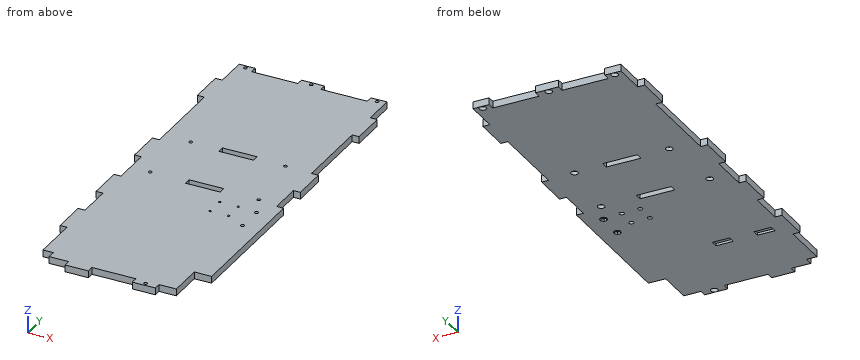
```python
from build123d import *

# Parameters (mm, degrees)
BOSS_EXTRU_1_DEPTH      = 6
ESQUISSE2_R             = 1.5
ESQUISSE2_W             = 30
ESQUISSE2_H             = 6
ENL_V_MAT_EXTRU_1_DEPTH = 226.720818795
ESQUISSE5_R             = 2.995
ENL_V_MAT_EXTRU_2_DEPTH = 3
ESQUISSE6_R             = 1.005
ENL_V_MAT_EXTRU_3_DEPTH = 226.720818795
ESQUISSE7_R             = 2
ENL_V_MAT_EXTRU_4_DEPTH = 2
ESQUISSE8_W             = 15
ESQUISSE8_H             = 30
ESQUISSE8_W_2           = 9
ESQUISSE8_H_2           = 7
ENL_V_MAT_EXTRU_5_DEPTH = 226.720818795
ESQUISSE13_R            = 1.6
ENL_V_MAT_EXTRU_7_DEPTH = 6
ESQUISSE14_W            = 15
ESQUISSE14_H            = 6
ESQUISSE14_R            = 1.6
ENL_V_MAT_EXTRU_8_DEPTH = 2


with BuildPart() as part:
    # Esquisse1 → Boss.-Extru.1 (new body)
    with BuildSketch(Plane.XY):
        Polygon((-67.628238976, -36.290343107), (-67.628238976, -70.290343107), (-73.628238976, -70.290343107), (-73.628238976, -100.290343107), (-67.628238976, -100.290343107), (-67.628238976, -130.290343107), (-73.628238976, -130.290343107), (-73.628238976, -160.290343107), (-67.628238976, -160.290343107), (-67.628238976, -207.290343107), (-41.628238976, -207.290343107), (-41.628238976, -213.290343107), (-21.628238976, -213.290343107), (-21.628238976, -207.290343107), (16.371761024, -207.290343107), (16.371761024, -213.290343107), (36.371761024, -213.290343107), (36.371761024, -207.290343107), (66.371761024, -207.290343107), (66.371761024, -57.290343107), (60.371761024, -57.290343107), (60.371761024, -29.290343107), (66.371761024, -29.290343107), (66.371761024, 0.709656893), (60.371761024, 0.709656893), (60.371761024, 68.709656893), (66.371761024, 68.709656893), (66.371761024, 98.709656893), (60.371761024, 98.709656893), (60.371761024, 126.709656893), (46.371761024, 126.709656893), (46.371761024, 120.709656893), (6.371761024, 120.709656893), (6.371761024, 126.709656893), (-13.628238976, 126.709656893), (-13.628238976, 120.709656893), (-53.628238976, 120.709656893), (-53.628238976, 126.709656893), (-67.628238976, 126.709656893), (-67.628238976, 98.709656893), (-73.628238976, 98.709656893), (-73.628238976, 68.709656893), (-67.628238976, 68.709656893), (-67.628238976, -6.290343107), (-73.628238976, -6.290343107), (-73.628238976, -36.290343107), align=None)
    extrude(amount=BOSS_EXTRU_1_DEPTH)

    # Esquisse2 → Enlèv. mat.-Extru.1 (cut, through all)
    with BuildSketch(Plane.XY.offset(6)):
        with Locations((-44.628238976, 1.709656893)):
            Circle(ESQUISSE2_R)
        with Locations((37.371761024, 1.709656893)):
            Circle(ESQUISSE2_R)
        with Locations((43.371761024, -54.290343107)):
            Circle(ESQUISSE2_R)
        with Locations((-50.628238976, -54.290343107)):
            Circle(ESQUISSE2_R)
        with Locations((-3.628238976, 123.709656893)):
            Circle(ESQUISSE2_R)
        with Locations((-60.628238976, 123.709656893)):
            Circle(ESQUISSE2_R)
        with Locations((53.371761024, 123.709656893)):
            Circle(ESQUISSE2_R)
        with Locations((26.371761024, -210.290343107)):
            Circle(ESQUISSE2_R)
        with Locations((-3.628238976, 1.709656893)):
            Rectangle(ESQUISSE2_W, ESQUISSE2_H)
        with Locations((-3.628238976, -54.290343107)):
            Rectangle(ESQUISSE2_W, ESQUISSE2_H)
    extrude(amount=-ENL_V_MAT_EXTRU_1_DEPTH, mode=Mode.SUBTRACT)

    # Esquisse5 → Enlèv. mat.-Extru.2 (cut)
    with BuildSketch(Plane(origin=(0, 0, 0), x_dir=(-1, 0, 0), z_dir=(0, 0, -1))):
        with Locations((-43.371761024, -54.290343107)):
            Circle(ESQUISSE5_R)
        with Locations((50.628238976, -54.290343107)):
            Circle(ESQUISSE5_R)
        with Locations((44.628238976, 1.709656893)):
            Circle(ESQUISSE5_R)
        with Locations((-37.371761024, 1.709656893)):
            Circle(ESQUISSE5_R)
        with Locations((-53.371761024, 123.709656893)):
            Circle(ESQUISSE5_R)
        with Locations((3.628238976, 123.709656893)):
            Circle(ESQUISSE5_R)
        with Locations((60.628238976, 123.709656893)):
            Circle(ESQUISSE5_R)
        with Locations((-26.371761024, -210.290343107)):
            Circle(ESQUISSE5_R)
    extrude(amount=-ENL_V_MAT_EXTRU_2_DEPTH, mode=Mode.SUBTRACT)

    # Esquisse6 → Enlèv. mat.-Extru.3 (cut, through all)
    with BuildSketch(Plane(origin=(0, 0, 0), x_dir=(-1, 0, 0), z_dir=(0, 0, -1))):
        with Locations((-34.371761024, -71.290343107)):
            Circle(ESQUISSE6_R)
        with Locations((-18.361761024, -71.290343107)):
            Circle(ESQUISSE6_R)
        with Locations((-34.371761024, -87.290343107)):
            Circle(ESQUISSE6_R)
        with Locations((-18.361761024, -87.290343107)):
            Circle(ESQUISSE6_R)
    extrude(amount=-ENL_V_MAT_EXTRU_3_DEPTH, mode=Mode.SUBTRACT)

    # Esquisse7 → Enlèv. mat.-Extru.4 (cut)
    with BuildSketch(Plane(origin=(0, 0, 0), x_dir=(-1, 0, 0), z_dir=(0, 0, -1))):
        with Locations((-34.371761024, -71.290343107)):
            Circle(ESQUISSE7_R)
        with Locations((-18.361761024, -71.290343107)):
            Circle(ESQUISSE7_R)
        with Locations((-18.361761024, -87.290343107)):
            Circle(ESQUISSE7_R)
        with Locations((-34.371761024, -87.290343107)):
            Circle(ESQUISSE7_R)
    extrude(amount=-ENL_V_MAT_EXTRU_4_DEPTH, mode=Mode.SUBTRACT)

    # Esquisse8 → Enlèv. mat.-Extru.5 (cut, through all)
    with BuildSketch(Plane(origin=(0, 0, 0), x_dir=(-1, 0, 0), z_dir=(0, 0, -1))):
        with Locations((-58.871761024, -192.290343107)):
            Rectangle(ESQUISSE8_W, ESQUISSE8_H)
        with Locations((63.128238976, -203.790343107)):
            Rectangle(ESQUISSE8_W_2, ESQUISSE8_H_2)
    extrude(amount=-ENL_V_MAT_EXTRU_5_DEPTH, mode=Mode.SUBTRACT)

    # Esquisse13 → Enlèv. mat.-Extru.7 (cut)
    with BuildSketch(Plane(origin=(0, 0, 0), x_dir=(-1, 0, 0), z_dir=(0, 0, -1))):
        with Locations((-50.971761024, -72.790343107)):
            Circle(ESQUISSE13_R)
        with Locations((-50.971761024, -95.790343107)):
            Circle(ESQUISSE13_R)
    extrude(amount=-ENL_V_MAT_EXTRU_7_DEPTH, mode=Mode.SUBTRACT)

    # Esquisse14 → Enlèv. mat.-Extru.8 (cut)
    # profile 1 of 4: a face of its own
    with BuildSketch(Plane(origin=(0, 0, 0), x_dir=(-1, 0, 0), z_dir=(0, 0, -1))):
        with Locations((50.128238976, -146.290343107)):
            Rectangle(ESQUISSE14_W, ESQUISSE14_H)
    # profile 2 of 4: a face of its own
    with BuildSketch(Plane(origin=(0, 0, 0), x_dir=(-1, 0, 0), z_dir=(0, 0, -1))):
        Polygon((-52.214401711, -69.790343107), (-49.729120337, -69.790343107), (-47.971761024, -71.54770242), (-47.971761024, -74.032983794), (-49.729120337, -75.790343107), (-52.214401711, -75.790343107), (-53.971761024, -74.032983794), (-53.971761024, -71.54770242), align=None)
        with Locations((-50.971761024, -72.790343107)):
            Circle(ESQUISSE14_R, mode=Mode.SUBTRACT)
    # profile 3 of 4: a face of its own
    with BuildSketch(Plane(origin=(0, 0, 0), x_dir=(-1, 0, 0), z_dir=(0, 0, -1))):
        with Locations((14.128238976, -146.290343107)):
            Rectangle(ESQUISSE14_W, ESQUISSE14_H)
    # profile 4 of 4: a face of its own
    with BuildSketch(Plane(origin=(0, 0, 0), x_dir=(-1, 0, 0), z_dir=(0, 0, -1))):
        Polygon((-47.971761024, -94.54770242), (-49.729120337, -92.790343107), (-52.214401711, -92.790343107), (-53.971761024, -94.54770242), (-53.971761024, -97.032983794), (-52.214401711, -98.790343107), (-49.729120337, -98.790343107), (-47.971761024, -97.032983794), align=None)
        with Locations((-50.971761024, -95.790343107)):
            Circle(ESQUISSE14_R, mode=Mode.SUBTRACT)
    extrude(amount=-ENL_V_MAT_EXTRU_8_DEPTH, mode=Mode.SUBTRACT)


solid = part.part
```
For this review, take the finished solid that the model builds, in its own axes (mm). Coordinates: 2 decimals unless noted, no trailing zeros. Write each loop counter-clockwise with the first axis right and the second up, starting at its lowest first coordinate (ties: lowest second). Pieces come first, ordered by that corner, then holes. Notation, with made-up numbers: (21.25, 77.25) -> (62.25, 77.25) arc R16 cw to (62.25, 87.25) -> close; hole circle Ø5 at (-34.5, -17). An arc over 180 degrees is marked (long way). Put each result on its own line as item: value.
Q1. Take a section at C-C, the plane y = -114.5. State the section outline as (x, z) points.
From the geometry:
outline: (-67.63, 0) -> (66.37, 0) -> (66.37, 6) -> (-67.63, 6) -> close
Q2. Take a section at B-B, the plane z = 4.75. Count the separate pieces of the cut face and the enclosed holes in it, then the cut area to 3 significant figures.
From the geometry:
separate pieces: 1
enclosed holes: 16
area: 43,500 mm2
Q3. Take a section at A-A, the plane y = 8.5. State the section outline as (x, z) points.
From the geometry:
outline: (-67.63, 0) -> (60.37, 0) -> (60.37, 6) -> (-67.63, 6) -> close
Q4. Clearance check with flat-ended pins moving along their axes: pin 1 Ø5 at (x, y) = (-60.63, 123.71) entering from -Z; pin 2 Ø1.2 at (x, y) = (35.5, -88) entering from -Z; pin 3 Ø1.2 at (x, y) = (34.37, -71.29) entering from +Z; pin 4 Ø3 at (y, z) = (0.5, 4.5) entering from -X. State where each tip first meets the part, or that it passes through.
From the geometry:
pin 1: stops at z = 3
pin 2: stops at z = 2
pin 3: passes through
pin 4: stops at x = -67.63
Q5. Wall thickness on L1, parallel to Y at x = -2, z = 3.4; L2, parallel to Y at x = -55, z = 1.3; L3, parallel to Y at x = -42, z = 0.45: over which ranges is each line inside the solid? List them lowest first.
From the geometry:
L1: y = -207.29 to -57.29, -51.29 to -1.29, 4.71 to 126.71
L2: y = -207.29 to -149.29, -143.29 to 126.71
L3: y = -207.29 to 0.27, 3.15 to 120.71
